from build123d import *

# Parameters (mm, degrees)
SKETCH1_R         = 40.5
SKETCH1_R_2       = 7.5
EXTRUDE_1_4_DEPTH = 10
SKETCH2_R         = 2.75
M5_THROUGH_DEPTH  = 10
CIRPATTERN5_COUNT = 8


with BuildPart() as part:
    # Sketch1 → 1/4 (new body)
    with BuildSketch(Plane.XY):
        Circle(SKETCH1_R)
        Circle(SKETCH1_R_2, mode=Mode.SUBTRACT)
    extrude(amount=EXTRUDE_1_4_DEPTH)

    # Sketch2 → M5_through (cut)
    with BuildSketch(Plane.XY):
        with Locations((0, 15)):
            Circle(SKETCH2_R)
    m5_through = extrude(amount=M5_THROUGH_DEPTH, mode=Mode.SUBTRACT)

    # CirPattern5: M5_through ×8 about axis
    cirpattern5_axis = Axis((0, 0, 0), (0, 0, 1))
    for i in range(1, CIRPATTERN5_COUNT):
        add(m5_through.rotate(cirpattern5_axis, i * 360 / CIRPATTERN5_COUNT), mode=Mode.SUBTRACT)


solid = part.part
Input: part model. Units: mm. Frame: model coordinates. Give positions to 0.01 mm unless a question says otherwise; leave off trailing zeros. Loops run counter-clockwise (first coordinate to the right, second up) from the corner with the lowest first, then second, coordinate; pieces in that order, holes last. Notation, with made-up numbers: (41.25, -20.5) -> (91.25, -20.5) arc R35 ccw to (91.25, 12.5) -> close; hole circle Ø3 at (-6, 26). An arc over 180 degrees is marked (long way). Answer as a JSON object with one key per item and string values. Group by question number.
Item 1: Line query: probe 1 along Y at (x, z) = (0, 4.5); probe 2 along Y at (x, z) = (-15.5, 0.5); probe 3 along Y at (x, z) = (-12.5, 8). Output: solid intervals per line, ascending.
Item 2: Cut plane A-A, the plane y = 0. Return the cut outline in (x, z).
Item 3: Cut plane C-C, the plane z = 5.75. State how many separate pieces and enclosed holes the cut face has, and give its area (3 significant figures).
Item 4: Pin query (flat end, axial travel): P1, Ø4.5, axis at x = 10.61, y = -10.61, coming from the +Z side; P2, Ø5, axis at x = 23, z = 7, coming from the +Y side; P3, Ø1.5, axis at y = 16, z = 7, coming from the +X side; P4, Ø2, axis at x = 2.5, z = 6, coming from the +Y side. Return the tip coordinate at first contact, or that it passes through.
Item 5: Cut plane B-B, the plane x = -15. Return the cut outline in (y, z), and give its area (3 significant figures).
Item 6: Cut plane D-D, the plane y = 10.5. Return the cut outline in (x, z).
Item 7: Pull-direction query (Y, two-part tool) for faces 1 (the cylindrical face through (8.287, 9.13, 4.93)), 2 (the flat face through (-1, -8, 0)), 3 (the cylindrical face through (21.77, 34.15, 4.93)); classes: released by +Y, released by -Y, zero draft, split by the parting line, or undercut.
Checks:
{
 "1": {"probe 1": "y = -40.5 to -17.75, -12.25 to -7.5, 7.5 to 12.25, 17.75 to 40.5", "probe 2": "y = -37.42 to -2.7, 2.7 to 37.42", "probe 3": "y = -38.52 to -12.6, -8.61 to -1.15, 1.15 to 8.61, 12.6 to 38.52"},
 "2": {"outline": "(-40.5, 0) -> (-17.75, 0) -> (-17.75, 10) -> (-40.5, 10) -> close; (-12.25, 0) -> (-7.5, 0) -> (-7.5, 10) -> (-12.25, 10) -> close; (7.5, 0) -> (12.25, 0) -> (12.25, 10) -> (7.5, 10) -> close; (17.75, 0) -> (40.5, 0) -> (40.5, 10) -> (17.75, 10) -> close"},
 "3": {"separate pieces": "1", "enclosed holes": "9", "area": "4,790 mm²"},
 "4": {"P1": "passes through", "P2": "stops at y = 34.93", "P3": "stops at x = 37.52", "P4": "stops at y = 40.47"},
 "5": {"outline": "(-37.62, 0) -> (-2.75, 0) -> (-2.75, 10) -> (-37.62, 10) -> close; (2.75, 0) -> (37.62, 0) -> (37.62, 10) -> (2.75, 10) -> close", "area": "697 mm²"},
 "6": {"outline": "(-39.12, 0) -> (-13.35, 0) -> (-13.35, 10) -> (-39.12, 10) -> close; (-7.86, 0) -> (7.86, 0) -> (7.86, 10) -> (-7.86, 10) -> close; (13.35, 0) -> (39.12, 0) -> (39.12, 10) -> (13.35, 10) -> close"},
 "7": {"face 1": "undercut", "face 2": "zero draft", "face 3": "split by the parting line"}
}
